```python
from build123d import *

# Parameters (mm, degrees)
F0_W      = 1219.2
F0_H      = 1219.2
F1_DEPTH  = 850.9
F2_R      = 152.4
F3_DEPTH  = 304.8
F4_R      = 285.75
F5_DEPTH  = 152.4
F7_DEPTH  = 1016
F8_W      = 1219.2
F8_H      = 1219.2
F9_DEPTH  = 152.4
F10_W     = 203.2
F10_H     = 304.8
F11_DEPTH = 177.8
F12_R     = 50.8
F13_DEPTH = 622.3
F15_DEPTH = 304.8
F16_R     = 50.8
F17_DEPTH = 304.8


with BuildPart() as f1:
    # F0 (on Top) → F1 (new body)
    with BuildSketch(Plane.XY):
        Rectangle(F0_W, F0_H)
    extrude(amount=F1_DEPTH)

    # F2 (on face) → F3 (cut)
    with BuildSketch(Plane.XY.offset(850.9)):
        Circle(F2_R)
    extrude(amount=-F3_DEPTH, mode=Mode.SUBTRACT)

    # F4 (on face) → F5 (cut)
    with BuildSketch(Plane.XY.offset(850.9)):
        Circle(F4_R)
    extrude(amount=-F5_DEPTH, mode=Mode.SUBTRACT)

    # F6 (on face) → F7 (join)
    with BuildSketch(Plane.XY.offset(850.9)):
        Polygon((-609.6, -609.6), (609.6, -609.6), (609.6, -457.2), (-457.2, -457.2), (-457.2, 457.2), (609.6, 457.2), (609.6, 609.6), (-609.6, 609.6), align=None)
    extrude(amount=F7_DEPTH)

    # F8 (on face) → F9 (join)
    with BuildSketch(Plane.XY.offset(1866.9)):
        Rectangle(F8_W, F8_H)
    extrude(amount=F9_DEPTH)

    # F10 (on face) → F11 (join)
    with BuildSketch(Plane.XY.offset(2019.3)):
        Rectangle(F10_W, F10_H)
    extrude(amount=F11_DEPTH)

    # F12 (on face) → F13 (cut)
    with BuildSketch(Plane.YZ.offset(101.6)):
        with Locations((0, 2108.2)):
            Circle(F12_R)
    extrude(amount=-F13_DEPTH, mode=Mode.SUBTRACT)

    # F15 (add): a face of the model
    f15_faces = [f1.faces().sort_by_distance(p)[0] for p in [
        (101.6, -148.8713192267, 2108.2),
    ]]
    extrude(f15_faces, amount=-F15_DEPTH)

    # F16 (on face) → F17 (cut)
    with BuildSketch(Plane.XY.offset(2019.3)):
        with Locations((374.4671290531, 0)):
            Circle(F16_R)
    extrude(amount=-F17_DEPTH, mode=Mode.SUBTRACT)


solid = f1.part
```
Geometry check sheet. Reference: the model listing, model coordinates, mm. A direction names the side the tool comes from. Round coordinates to 2 decimals unless told otherwise and drop trailing zeros. Loops run counter-clockwise (first coordinate to the right, second up) from the corner with the lowest first, then second, coordinate; pieces in that order, holes last. Notation, with made-up numbers: (40, 73) - (92, 73) arc R26 ccw to (92, 104) - close; hole circle Ø3 at (17, 47.25). An arc over 180 degrees is marked (long way). Write item = value, one per line. Start each with the question number.
1. Mould release check, pull along Y, two halves, no side actions. Record for faces 1 (the face through (-9, -609.6, 996)), 2 (the face through (-9, 609.6, 996)), 3 (the face through (-120.94, -92.73, 623.37)), 4 (the face through (-457.2, -6, 1352)): released by +Y, released by -Y, zero draft, split by the parting line, or undercut.
2. Set-up check for faces 5 (the face through (101.6, -36, 2067)), 6 (the face through (69, 457.2, 1352)), 7 (the face through (123, -123, 698.5)), 8 (the face through (-49, 152.4, 2107)): record each of +Z, -Z, +X, -X, +Y, -Y from which the full face is reachable in a straight line by a thin tool's end or side.
3. Thickness scan on line 1 (Z direction, x = -25, y = 0); line 2 (Z direction, x = 171, y = -96.5); line 3 (Z direction, x = -10, y = -136). Record the ranges inside material, lowest first.
4. Section check A-A on z = 2108.2. Enter the section's corners in (x, y), then the cut area to 3 significant figures.
5. Section check D-D on z = 944. Enter the section's corners in (x, y).
6. Section check B-B on x = 0. Enter the section's corners in (y, z), then the cut area to 3 significant figures.
7. Section check C-C on y = 0. Enter the section's corners in (x, z), then the cut area to 3 significant figures.
8. Depth check by flat-ended pin: pin 1 (8 mm diameter, centred on x = 188, y = 122, fed in from +Z); pin 2 (1 mm diameter, centred on y = 186.5, z = 1712.5, fed in from +X). Enter the tip coordinate at first touch or a pass-through.
Working result:
q1.face_1 = released by -Y
q1.face_2 = released by +Y
q1.face_3 = undercut
q1.face_4 = undercut
q2.face_5 = +Z, +X, +Y, -Y
q2.face_6 = +X
q2.face_7 = none
q2.face_8 = +Z, +X, -X, +Y
q3.line_1 = 0 to 546.1, 1866.9 to 2057.4, 2159 to 2197.1
q3.line_2 = 0 to 698.5, 1866.9 to 2019.3
q3.line_3 = 0 to 546.1, 1866.9 to 2197.1
q4.outline = (-203.2, -152.4) - (101.6, -152.4) - (101.6, -50.8) - (-203.2, -50.8) - close; (-203.2, 50.8) - (101.6, 50.8) - (101.6, 152.4) - (-203.2, 152.4) - close
q4.area = 61,900 mm^2
q5.outline = (-609.6, -609.6) - (609.6, -609.6) - (609.6, -457.2) - (-457.2, -457.2) - (-457.2, 457.2) - (609.6, 457.2) - (609.6, 609.6) - (-609.6, 609.6) - close
q6.outline = (-609.6, 0) - (609.6, 0) - (609.6, 2019.3) - (152.4, 2019.3) - (152.4, 2197.1) - (-152.4, 2197.1) - (-152.4, 2019.3) - (-609.6, 2019.3) - close; hole (-457.2, 850.9) - (-285.75, 850.9) - (-285.75, 698.5) - (-152.4, 698.5) - (-152.4, 546.1) - (152.4, 546.1) - (152.4, 698.5) - (285.75, 698.5) - (285.75, 850.9) - (457.2, 850.9) - (457.2, 1866.9) - (-457.2, 1866.9) - close; hole circle Ø101.6 at (0, 2108.2)
q6.area = 1,450,000 mm^2
q7.outline = (-609.6, 0) - (609.6, 0) - (609.6, 850.9) - (285.75, 850.9) - (285.75, 698.5) - (152.4, 698.5) - (152.4, 546.1) - (-152.4, 546.1) - (-152.4, 698.5) - (-285.75, 698.5) - (-285.75, 850.9) - (-457.2, 850.9) - (-457.2, 1866.9) - (323.67, 1866.9) - (323.67, 2019.3) - (101.6, 2019.3) - (101.6, 2057.4) - (-203.2, 2057.4) - (-203.2, 2019.3) - (-609.6, 2019.3) - close; (-203.2, 2159) - (101.6, 2159) - (101.6, 2197.1) - (-203.2, 2197.1) - close; (425.27, 1866.9) - (609.6, 1866.9) - (609.6, 2019.3) - (425.27, 2019.3) - close
q7.area = 1,250,000 mm^2
q8.pin_1 = 2019.3
q8.pin_2 = -457.2
